Part model, mm, in its own coordinate system. A direction names the side the tool comes from. Round coordinates to 2 decimals unless told otherwise and drop trailing zeros. Loops run counter-clockwise (first coordinate to the right, second up) from the corner with the lowest first, then second, coordinate; pieces in that order, holes last.
Autodesk Fusion 360 part; units mm, degrees
sketch "Skizze1" plane through (0, 0, 0) normal (0, 0, 1) x (1, 0, 0)
  line L0 (33.75, -19.75) -> (-33.75, -19.75)
  line L1 (-33.75, -19.75) -> (-33.75, 19.75)
  line L2 (-33.75, 19.75) -> (33.75, 19.75)
  line L3 (33.75, 19.75) -> (33.75, -19.75)
  line L4 (33.75, -19.75) -> (-33.75, 19.75) construction
  line L5 (-33.75, -19.75) -> (33.75, 19.75) construction
  dimension "d1" = 67.5
  dimension "d2" = 39.5
extrude "Extrusion1" add sketch "Skizze1" along normal blind 6
sketch "Skizze2" plane through (0, 0, 6) normal (0, 0, 1) x (-1, 0, 0)
  line L0 (-33.75, -19.75) -> (33.75, -19.75)
  line L1 (33.75, -19.75) -> (33.75, 19.75)
  line L2 (33.75, 19.75) -> (-33.75, 19.75)
  line L3 (-33.75, 19.75) -> (-33.75, -19.75)
  line L4 (31.25, 17.25) -> (-31.25, 17.25)
  line L5 (-31.25, 17.25) -> (-31.25, -17.25)
  line L6 (-31.25, -17.25) -> (31.25, -17.25)
  line L7 (31.25, -17.25) -> (31.25, 17.25)
  line L8 (31.25, 17.25) -> (-31.25, -17.25) construction
  line L9 (-31.25, 17.25) -> (31.25, -17.25) construction
  dimension "d5" = 34.5
  dimension "d6" = 62.5
extrude "Extrusion2" cut sketch "Skizze2" against normal blind 1 contours L4 L5 L6 L7
sketch "Skizze3" plane through (0, 0, 5) normal (0, 0, 1) x (-1, 0, 0)
  line L0 (31.25, -17.25) -> (31.25, 17.25)
  line L1 (31.25, 17.25) -> (-31.25, 17.25)
  line L2 (-31.25, 17.25) -> (-31.25, -17.25)
  line L3 (-31.25, -17.25) -> (31.25, -17.25)
  line L4 (29.75, -15.75) -> (-29.75, -15.75)
  line L5 (-29.75, -15.75) -> (-29.75, 15.75)
  line L6 (-29.75, 15.75) -> (29.75, 15.75)
  line L7 (29.75, 15.75) -> (29.75, -15.75)
  line L8 (29.75, -15.75) -> (-29.75, 15.75) construction
  line L9 (-29.75, -15.75) -> (29.75, 15.75) construction
  line L10 (28.605, -14.605) -> (-0.605, -14.605) construction
  line L11 (-0.605, -14.605) -> (-0.605, 14.605) construction
  line L12 (-0.605, 14.605) -> (28.605, 14.605) construction
  line L13 (28.605, 14.605) -> (28.605, -14.605) construction
  line L14 (31.25, -17.25) -> (28.605, -14.605) construction
  line L15 (31.25, 17.25) -> (28.605, 14.605) construction
  line L16 (28.605, -11.605) -> (29.75, -11.605)
  line L17 (25.605, -14.605) -> (25.605, -15.75)
  line L18 (28.605, 11.605) -> (29.75, 11.605)
  line L19 (25.605, 14.605) -> (25.605, 15.75)
  arc A0 (28.605, -11.605) -> (25.605, -14.605) centre (28.605, -14.605) ccw
  arc A1 (25.605, 14.605) -> (28.605, 11.605) centre (28.605, 14.605) ccw
  line L20 (2.395, 14.605) -> (2.395, 15.75)
  line L21 (-3.605, 14.605) -> (-3.605, 15.75)
  line L22 (2.395, -14.605) -> (2.395, -15.75)
  line L23 (-3.605, -14.605) -> (-3.605, -15.75)
  arc A2 (2.395, -14.605) -> (-3.605, -14.605) centre (-0.605, -14.605) ccw
  arc A3 (-3.605, 14.605) -> (2.395, 14.605) centre (-0.605, 14.605) ccw
  dimension "d9" = 1.5
  dimension "d10" = 1.5
  dimension "d13" = 29.21
  dimension "d14" = 29.21
  dimension "d15" = 6
extrude "Extrusion3" cut sketch "Skizze3" against normal up to surface (3.5 mm away) contours L4 L5 L6 L7 L16 L17 L18 L19 A0 A1 L20 L21 L22 L23 A2 A3
sketch "Skizze4" plane through (0, 0, 5) normal (0, 0, 1) x (-1, 0, 0)
  line L0 (2.395, 14.605) -> (2.395, 15.75)
  line L1 (2.395, 15.75) -> (25.605, 15.75)
  line L2 (25.605, 15.75) -> (25.605, 14.605)
  arc A0 (25.605, 14.605) -> (28.605, 11.605) centre (28.605, 14.605) ccw
  line L3 (28.605, 11.605) -> (29.75, 11.605)
  line L4 (29.75, 11.605) -> (29.75, -11.605)
  line L5 (29.75, -11.605) -> (28.605, -11.605)
  arc A1 (28.605, -11.605) -> (25.605, -14.605) centre (28.605, -14.605) ccw
  line L6 (25.605, -14.605) -> (25.605, -15.75)
  line L7 (25.605, -15.75) -> (2.395, -15.75)
  line L8 (2.395, -15.75) -> (2.395, -14.605)
  arc A2 (2.395, -14.605) -> (-3.605, -14.605) centre (-0.605, -14.605) ccw
  line L9 (-3.605, -14.605) -> (-3.605, -15.75)
  line L10 (-3.605, -15.75) -> (-29.75, -15.75)
  line L11 (-29.75, -15.75) -> (-29.75, 15.75)
  line L12 (-29.75, 15.75) -> (-3.605, 15.75)
  line L13 (-3.605, 15.75) -> (-3.605, 14.605)
  arc A3 (-3.605, 14.605) -> (2.395, 14.605) centre (-0.605, 14.605) ccw
  line L14 (31.25, -17.25) -> (31.25, 17.25)
  line L15 (31.25, 17.25) -> (-31.25, 17.25)
  line L16 (-31.25, 17.25) -> (-31.25, -17.25)
  line L17 (-31.25, -17.25) -> (31.25, -17.25)
  circle A4 centre (28.605, -14.605) radius 1.15
  circle A5 centre (-0.605, -14.605) radius 1.15
  circle A6 centre (28.605, 14.605) radius 1.15
  circle A7 centre (-0.605, 14.605) radius 1.15
  dimension "d16" = 2.3
extrude "Extrusion4" cut sketch "Skizze4" against normal through all contours A4 | A5 | A6 | A7
sketch "Skizze5" plane through (0, 0, 0) normal (0, 0, -1) x (1, 0, 0)
  circle A0 centre (0.605, -14.605) radius 1.15
  circle A1 centre (-28.605, 14.605) radius 1.15
  circle A2 centre (-28.605, -14.605) radius 1.15
  circle A3 centre (0.605, 14.605) radius 1.15
  line L0 (-33.75, -19.75) -> (33.75, -19.75)
  line L1 (33.75, -19.75) -> (33.75, 19.75)
  line L2 (33.75, 19.75) -> (-33.75, 19.75)
  line L3 (-33.75, 19.75) -> (-33.75, -19.75)
  line L4 (-27.3926, 12.505) -> (-26.1801, 14.605)
  line L5 (-26.1801, 14.605) -> (-27.3926, 16.705)
  line L6 (-27.3926, 16.705) -> (-29.8174, 16.705)
  line L7 (-29.8174, 16.705) -> (-31.0299, 14.605)
  line L8 (-31.0299, 14.605) -> (-29.8174, 12.505)
  line L9 (-29.8174, 12.505) -> (-27.3926, 12.505)
  circle A4 centre (-28.605, 14.605) radius 1.15
  line L10 (-29.8174, -12.505) -> (-31.0299, -14.605)
  line L11 (-31.0299, -14.605) -> (-29.8174, -16.705)
  line L12 (-29.8174, -16.705) -> (-27.3926, -16.705)
  line L13 (-27.3926, -16.705) -> (-26.1801, -14.605)
  line L14 (-26.1801, -14.605) -> (-27.3926, -12.505)
  line L15 (-27.3926, -12.505) -> (-29.8174, -12.505)
  line L16 (1.8174, 12.505) -> (3.0299, 14.605)
  line L17 (3.0299, 14.605) -> (1.8174, 16.705)
  line L18 (1.8174, 16.705) -> (-0.6074, 16.705)
  line L19 (-0.6074, 16.705) -> (-1.8199, 14.605)
  line L20 (-1.8199, 14.605) -> (-0.6074, 12.505)
  line L21 (-0.6074, 12.505) -> (1.8174, 12.505)
  line L22 (-0.6074, -12.505) -> (-1.8199, -14.605)
  line L23 (-1.8199, -14.605) -> (-0.6074, -16.705)
  line L24 (-0.6074, -16.705) -> (1.8174, -16.705)
  line L25 (1.8174, -16.705) -> (3.0299, -14.605)
  line L26 (3.0299, -14.605) -> (1.8174, -12.505)
  line L27 (1.8174, -12.505) -> (-0.6074, -12.505)
  circle A5 centre (0.605, -14.605) radius 1.15
  point P0 (-28.605, 14.605)
  point P1 (-28.605, -14.605)
  point P2 (0.605, 14.605)
  point P3 (0.605, -14.605)
  dimension "d18" = 4.2
extrude "Extrusion5" cut sketch "Skizze5" against normal blind 2.5 contours L4 L5 L6 L7 L8 L9 | L10 L11 L12 L13 L14 L15 | L16 L17 L18 L19 L20 L21 | L22 L23 L24 L25 L26 L27
equation "d10 = d9"
1) Tool access for faces 3 (the face through (-14, 15.75, 3)), 4 (the face through (-0.013, 13.635, 3.768)), 5 (the face through (-1.222, 15.64, 1.232)): list every direction of +Z, -Z, +X, -X, +Y, -Y with a clear straight run to the whole face (end or side of a thin tool).
Values:
face 3: +Z
face 4: +Z, -Z
face 5: -Z
2) Slice it at A-A, the plane z = 4.2. Give the cut face in (x, y) (3 decimals), then the cut area to 3 significant figures.
Values:
outline: (-33.75, -19.75) - (33.75, -19.75) - (33.75, 19.75) - (-33.75, 19.75) - close; hole circle Ø2.3 at (-28.605, -14.605); hole circle Ø2.3 at (-28.605, 14.605); hole (-29.75, -11.605) - (-28.605, -11.605) arc R3 cw to (-25.605, -14.605) - (-25.605, -15.75) - (-2.395, -15.75) - (-2.395, -14.605) arc R3 cw to (3.605, -14.605) - (3.605, -15.75) - (29.75, -15.75) - (29.75, 15.75) - (3.605, 15.75) - (3.605, 14.605) arc R3 cw to (-2.395, 14.605) - (-2.395, 15.75) - (-25.605, 15.75) - (-25.605, 14.605) arc R3 cw to (-28.605, 11.605) - (-29.75, 11.605) - close; hole circle Ø2.3 at (0.605, -14.605); hole circle Ø2.3 at (0.605, 14.605)
area: 848 mm2
3) Slice it at C-C, the plane y = 2. Give the cut face in (x, z), then the cut area to 3 significant figures.
Values:
outline: (-33.75, 0) - (33.75, 0) - (33.75, 6) - (31.25, 6) - (31.25, 5) - (29.75, 5) - (29.75, 1.5) - (-29.75, 1.5) - (-29.75, 5) - (-31.25, 5) - (-31.25, 6) - (-33.75, 6) - close
area: 134 mm2
4) Slice it at B-B, the plane x = 27.5. Give the cut face in (y, z).
Values:
outline: (-19.75, 0) - (19.75, 0) - (19.75, 6) - (17.25, 6) - (17.25, 5) - (15.75, 5) - (15.75, 1.5) - (-15.75, 1.5) - (-15.75, 5) - (-17.25, 5) - (-17.25, 6) - (-19.75, 6) - close
5) Wall check: line 1 along X through (y, z) = (1.5, 5.05); line 2 along X through (y, z) = (0, 2.4); line 3 along Y through (x, z) = (21, 2.2). Give the ranges that are in metal, low to high.
Values:
line 1: x = -33.75 to -31.25, 31.25 to 33.75
line 2: x = -33.75 to -29.75, 29.75 to 33.75
line 3: y = -19.75 to -15.75, 15.75 to 19.75
6) Drop flat-ended pins along their axis: pin 1 Ø1.8 at (x, y) = (0.605, -14.605) entering from -Z; pin 2 Ø3 at (x, y) = (17, -7) entering from +Z; pin 3 Ø2.5 at (x, y) = (0.605, 14.605) entering from +Z. Give the stop position or say it passes through.
Values:
pin 1: passes through
pin 2: stops at z = 1.5
pin 3: stops at z = 5
7) Mould opens along X. For faces 1 (the face through (2.432, -15.64, 1.232)), 2 (the face through (0, -19.75, 3)) say: released by +X, released by -X, zero draft, split by the parting line, or undercut.
Values:
face 1: undercut
face 2: zero draft
